CAD build for the part. Positions are in the model's coordinates, mm. A direction names the side the tool comes from. Give positions to 0.01 mm unless a question says otherwise; leave off trailing zeros. Write each loop counter-clockwise with the first axis right and the second up, starting at its lowest first coordinate (ties: lowest second). Pieces come first, ordered by that corner, then holes. Notation, with made-up numbers: M 3.25,11.25 L 25.25,11.25 A22 ccw 25.25,33.25 Z; hole C 17.5,53 d3. An arc over 180 degrees is marked long. One line per question, with ' | ' between items. Start each with the question number.
1. Which spindle directions (+Z, -Z, +X, -X, +Y, -Y) get a long thin tool onto all of the face, cutting with end or side? Do faces 1 (the face through (44.823, 27.535, 26.364)), 2 (the face through (5, 47, -38)), 3 (the face through (-35.79, 47.32, -14.89)). Say none if no direction does.
2. Cut at C-C, the plane y = 4.5. Write the cut outline in (x, z), then the cut area to 3 significant figures.
3. Cut at B-B, the plane y = 37. Count the separate pieces of the cut face and the enclosed holes in it, then the cut area to 3 significant figures.
4. Wall check: L1, parallel to Z at x = 0, y = 28; L2, parallel to Y at x = 41, z = 4; L3, parallel to X at y = 37, z = 0. Give the ranges that are in metal, low to high.
5. Flat gauge pins, fed straight in: pin 1 (3 mm diameter, centred on y = 35, z = -35.5, fed in from -X); pin 2 (12.5 mm diameter, centred on y = 53.5, z = 33.5, fed in from +X); pin 3 (8 mm diameter, centred on y = 26, z = 11.5, fed in from +X); pin 4 (24.5 mm diameter, centred on x = -36, z = 22, fed in from +Y). Where does each tip first touch, or does it go through?
6. Pull direction X, two halves, no side cores. Call faces 4 (the face through (-45.24, 27.53, 25.64)), 5 (the face through (45.24, 27.53, -25.64)), 6 (the face through (5, 47, 38)): released by +X, released by -X, zero draft, split by the parting line, or undercut.
7. Cut at A-A, the plane x = 0. Write the cut outline in (y, z).
```python
from build123d import *

# Parameters (mm, degrees)
BOSS_EXTRUDE1_DEPTH = 60
SKETCH2_R           = 25
CUT_EXTRUDE1_DEPTH  = 60
SKETCH3_W           = 10
SKETCH3_H           = 25
CUT_EXTRUDE2_DEPTH  = 40
CIRPATTERN1_COUNT   = 6


with BuildPart() as part:
    # Sketch1 → Boss-Extrude1 (new body)
    with BuildSketch(Plane(origin=(0, 0, 0), x_dir=(1, 0, 0), z_dir=(0, 1, 0))):
        Polygon((-60.044427996, 0), (-30.022213998, -52), (30.022213998, -52), (60.044427996, 0), (30.022213998, 52), (-30.022213998, 52), align=None)
    extrude(amount=BOSS_EXTRUDE1_DEPTH)

    # Sketch2 → Cut-Extrude1 (cut)
    with BuildSketch(Plane(origin=(0, 60, 0), x_dir=(1, 0, 0), z_dir=(0, 1, 0))):
        Circle(SKETCH2_R)
    extrude(amount=-CUT_EXTRUDE1_DEPTH, mode=Mode.SUBTRACT)

    # Sketch3 → Cut-Extrude2 (cut)
    with BuildSketch(Plane.XY.offset(52)):
        with Locations((0, 47.5)):
            Rectangle(SKETCH3_W, SKETCH3_H)
    cut_extrude2 = extrude(amount=-CUT_EXTRUDE2_DEPTH, mode=Mode.SUBTRACT)

    # CirPattern1: Cut-Extrude2 ×6 about axis
    cirpattern1_axis = Axis((0, 0, 0), (0, 1, 0))
    for i in range(1, CIRPATTERN1_COUNT):
        add(cut_extrude2.rotate(cirpattern1_axis, i * 360 / CIRPATTERN1_COUNT), mode=Mode.SUBTRACT)

    # Sketch4 → Cut-Revolve1 (revolve, cut)
    with BuildSketch(Plane.XY):
        with BuildLine():
            Line((40.044427996, 60), (60.044427996, 60))
            Line((60.044427996, 60), (60.044427996, 40))
            ThreePointArc((60.044427996, 40), (54.186563619, 54.142135624), (40.044427996, 60))
        make_face()
    revolve(axis=Axis((0, 0, 0), (0, 1, 0)), mode=Mode.SUBTRACT)


solid = part.part
```
Here are the results:
1) face 1: +Z, +X, +Y, -Y | face 2: +Z, -Z, +Y | face 3: +Y
2) outline: M -60.04,0 L -30.02,-52 L 30.02,-52 L 60.04,0 L 30.02,52 L -30.02,52 Z; hole C 0,0 d50 | area: 7,400 mm^2
3) separate pieces: 6 | enclosed holes: 0 | area: 5,770 mm^2
4) L1: -52 to -25, 25 to 52 | L2: 0 to 59.97 | L3: -60.04 to -25, 25 to 60.04
5) pin 1: x = -40.41 | pin 2: x = 42.53 | pin 3: x = 55.71 | pin 4: y = 60
6) face 4: released by -X | face 5: released by +X | face 6: undercut
7) outline: M 0,-52 L 35,-52 L 35,-25 L 0,-25 Z; M 0,25 L 35,25 L 35,52 L 0,52 Z
